Job drawing, mm, ordinate dimensions from the low corner. One solid piece. Round coordinates to 2 decimals unless told otherwise and drop trailing zeros. Write each loop counter-clockwise with the first axis right and the second up, starting at its lowest first coordinate (ties: lowest second). Pieces come first, ordered by that corner, then holes. Notation, with made-up numbers: (12.5, -32) -> (35.5, -32) arc R30 ccw to (35.5, -10) -> close; hole circle Ø11 at (36.25, 44). An arc over 180 degrees is marked (long way). Use CSV: the item, a comma, the result in double quotes. Start each with the question number.
(1) Probe line 1 (Y direction, x = 83.5, z = 8.5); line 2 (Z direction, x = 79, y = 22); line 3 (X direction, y = 24.5, z = 15.5). List the from-to ranges inside material, lowest first. Write a range as [from, to].
(2) Drop flat-ended pins along their axis: pin 1 (2 mm diameter, centred on y = 25.5, z = 16.5, fed in from -X); pin 2 (2.5 mm diameter, centred on x = 59.5, y = 25.5, fed in from -Z); pin 3 (12 mm diameter, centred on x = 44.5, z = 17, fed in from -Y); pin 4 (12 mm diameter, centred on x = 62.5, y = 21.5, fed in from -Z). Give the stop position or say it passes through.
(3) Saw through at C-C (z = 7). Give the cut face in (x, y).
(4) Saw through at B-B (y = 25.25). Give the cut face in (x, z).
(5) Two-plate mould, pull along Y, no slides. Class the marked faces 1, 2, 3 and 4: released by +Y, released by -Y, zero draft, split by the parting line, or undercut.
(6) Saw through at A-A (x = 78). Give the cut face in (y, z).
(7) Saw through at D-D (y = 15.25). Give the cut face in (x, z).
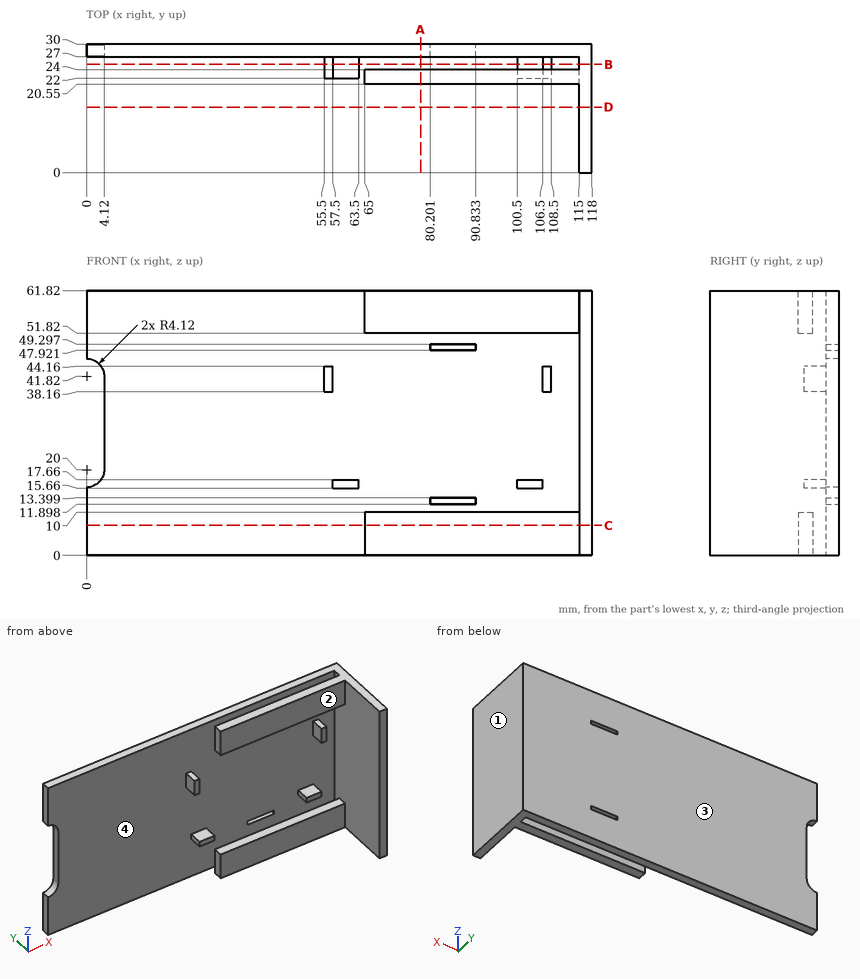
Answers:
1,line 1,"y = [20.55, 24], [27, 30]"
1,line 2,"z = [0, 10], [51.82, 61.82]"
1,line 3,"x = [115, 118]"
2,pin 1,"stops at x = 57.5"
2,pin 2,"stops at z = 15.66"
2,pin 3,"stops at y = 27"
2,pin 4,"stops at z = 0"
3,outline,"(0, 27) -> (115, 27) -> (115, 24) -> (65, 24) -> (65, 20.55) -> (115, 20.55) -> (115, 0) -> (118, 0) -> (118, 30) -> (0, 30) -> close"
4,outline,"(55.5, 38.16) -> (57.5, 38.16) -> (57.5, 44.16) -> (55.5, 44.16) -> close; (57.5, 15.66) -> (63.5, 15.66) -> (63.5, 17.66) -> (57.5, 17.66) -> close; (100.5, 15.66) -> (106.5, 15.66) -> (106.5, 17.66) -> (100.5, 17.66) -> close; (106.5, 38.16) -> (108.5, 38.16) -> (108.5, 44.16) -> (106.5, 44.16) -> close; (115, 0) -> (118, 0) -> (118, 61.82) -> (115, 61.82) -> close"
5,face 1,"zero draft"
5,face 2,"released by -Y"
5,face 3,"released by +Y"
5,face 4,"undercut"
6,outline,"(20.55, 0) -> (24, 0) -> (24, 10) -> (20.55, 10) -> close; (20.55, 51.82) -> (24, 51.82) -> (24, 61.82) -> (20.55, 61.82) -> close; (27, 0) -> (30, 0) -> (30, 61.82) -> (27, 61.82) -> close"
7,outline,"(115, 0) -> (118, 0) -> (118, 61.82) -> (115, 61.82) -> close"
